Work out the finished part from the listing and answer in its coordinate system (mm). A direction names the side the tool comes from. Round coordinates to 2 decimals unless told otherwise and drop trailing zeros. Order: outer loops, then holes, each group sorted by start corner. A loop starts at its lowest first (then second) coordinate and runs counter-clockwise, first axis right, second up. Notation, with made-up numbers: M 70,77.25 L 80,77.25 A7 cw 80,84.25 Z; hole C -40,-21 d9. An arc over 180 degrees is marked long. Return JSON: item names as keys, results as strings.
from build123d import *

# Parameters (mm, degrees)
BOSS_EXTRUDE1_DEPTH = 6.35


with BuildPart() as part:
    # Sketch1 → Boss-Extrude1 (new body)
    with BuildSketch(Plane(origin=(0, 0, 0), x_dir=(1, 0, 0), z_dir=(0, 1, 0))):
        Polygon((-28.0924, 15.5702), (-28.0924, 28.2702), (-19.289943879, 28.2702), (0, 8.980256121), (19.289943879, 28.2702), (28.0924, 28.2702), (28.0924, 15.5702), (21.7424, 15.5702), (21.7424, 12.762143879), (8.980256121, 0), (21.7424, -12.762143879), (21.7424, -15.5702), (28.0924, -15.5702), (28.0924, -28.2702), (19.289943879, -28.2702), (0, -8.980256121), (-19.289943879, -28.2702), (-28.0924, -28.2702), (-28.0924, -15.5702), (-21.7424, -15.5702), (-21.7424, -12.762143879), (-8.980256121, 0), (-21.7424, 12.762143879), (-21.7424, 15.5702), align=None)
        Polygon((6.286179285, 2.694076836), (2.694076836, 6.286179285), (17.9324, 21.524502448), (17.9324, 14.340297552), align=None, mode=Mode.SUBTRACT)
        Polygon((2.694076836, -6.286179285), (6.286179285, -2.694076836), (17.9324, -14.340297552), (17.9324, -21.524502448), align=None, mode=Mode.SUBTRACT)
        Polygon((-6.286179285, 2.694076836), (-2.694076836, 6.286179285), (-17.9324, 21.524502448), (-17.9324, 14.340297552), align=None, mode=Mode.SUBTRACT)
        Polygon((-6.286179285, -2.694076836), (-2.694076836, -6.286179285), (-17.9324, -21.524502448), (-17.9324, -14.340297552), align=None, mode=Mode.SUBTRACT)
    extrude(amount=BOSS_EXTRUDE1_DEPTH)


solid = part.part
Item 1: Find section C-C (z = 17.5). Determine the outline of the cut face in (x, y).
Output:
{"outline": "M -28.09,0 L -17.93,0 L -17.93,6.35 L -28.09,6.35 Z; M -13.91,0 L -8.52,0 L -8.52,6.35 L -13.91,6.35 Z; M 8.52,0 L 13.91,0 L 13.91,6.35 L 8.52,6.35 Z; M 17.93,0 L 28.09,0 L 28.09,6.35 L 17.93,6.35 Z"}
Item 2: Find section A-A (x = 7.5). Determine the outline of the cut face in (y, z), plus the area to 3 significant figures.
Output:
{"outline": "M 0,-16.48 L 6.35,-16.48 L 6.35,-11.09 L 0,-11.09 Z; M 0,-3.91 L 6.35,-3.91 L 6.35,3.91 L 0,3.91 Z; M 0,11.09 L 6.35,11.09 L 6.35,16.48 L 0,16.48 Z", "area": "118 mm^2"}
Item 3: The mould has two halves that part along Z. Classify faces 1 (the flat face through (-15.45, 3.13, 6.47)), 2 (the flat face through (24, 3, -28.27)), 3 (the flat face through (28.092, 3, -22)), 4 (the flat face through (-24, 3, 28.27)): pulls with the +Z half, pulls with the -Z half, needs draft (parallel to the pull), parting line crosses it, or undercut.
Output:
{"face 1": "undercut", "face 2": "pulls with the -Z half", "face 3": "needs draft", "face 4": "pulls with the +Z half"}
Item 4: Find section B-B (x = -21). Determine the outline of the cut face in (y, z).
Output:
{"outline": "M 0,-28.27 L 6.35,-28.27 L 6.35,-12.02 L 0,-12.02 Z; M 0,12.02 L 6.35,12.02 L 6.35,28.27 L 0,28.27 Z"}
Item 5: Each of these flat-tipped pins is pushed along its axis until it touches: pin 1 (2 mm diameter, centred on y = 1.5, z = -6.5, fed in from +X); pin 2 (3 mm diameter, centred on x = -3, y = 3, fed in from +Z); pin 3 (2 mm diameter, centred on y = 3.5, z = -13.5, fed in from +X). Where does it stop, or does it pass through?
Output:
{"pin 1": "stops at x = 16.48", "pin 2": "stops at z = 13.48", "pin 3": "stops at x = 21.74"}
Item 6: Find section D-D (z = -5.5). Determine the outline of the cut face in (x, y).
Output:
{"outline": "M -14.48,0 L -9.09,0 L -9.09,6.35 L -14.48,6.35 Z; M -3.48,0 L 3.48,0 L 3.48,6.35 L -3.48,6.35 Z; M 9.09,0 L 14.48,0 L 14.48,6.35 L 9.09,6.35 Z"}
Item 7: Which of the six approach directions +Z, -Z, +X, -X, +Y, -Y give full straight-line access (tool end or side, diameter ignored) to faces 5 (the flat face through (15.27, 3.13, 6.29)), 6 (the flat face through (9.78, 3.13, 18.76)), 7 (the flat face through (-12.19, 3.13, 8.6))?
Output:
{"face 5": "+X, +Y, -Y", "face 6": "+Z, +Y, -Y", "face 7": "+Y, -Y"}
Item 8: Consider line 1 along Z through (x, y) = (-10, 1.25); line 2 along Z through (x, y) = (17, 0.75); line 3 along X through (y, z) = (2.5, 3). Determine where each line is inside the solid, lowest interval first. Write a range as [from, to].
Output:
{"line 1": "z = [-18.98, -13.59], [-6.41, -1.02], [1.02, 6.41], [13.59, 18.98]", "line 2": "z = [-25.98, -20.59], [-13.41, -8.02], [8.02, 13.41], [20.59, 25.98]", "line 3": "x = [-11.98, -6.59], [-5.98, 5.98], [6.59, 11.98]"}
